Autodesk Inventor part; units mm, degrees
ref_plane "YZ Plane" through (0, 0, 0) normal (1, 0, 0) x (0, 1, 0)
ref_plane "XZ Plane" through (0, 0, 0) normal (0, 1, 0) x (-1, 0, 0)
ref_plane "XY Plane" through (0, 0, 0) normal (0, 0, 1) x (1, 0, 0)
sketch "Sketch1" plane through (0, 0, 0) normal (0, 1, 0) x (-1, 0, 0)
  line L0 (5, 7.5) -> (-5, 7.5)
  line L1 (-5, 7.5) -> (-5, -7.5)
  line L2 (-5, -7.5) -> (5, -7.5)
  line L3 (5, -7.5) -> (5, 7.5)
  point P0 (0, 0)
  dimension "d0" = 15
  dimension "d1" = 10
  dimension "d2" = 5
  dimension "d3" = 7.5
extrude "Extrusion1" add sketch "Sketch1" along normal blind 1.2
sketch "Sketch2" plane through (5, 0, 7.5) normal (1, 0, 0) x (0, 0, -1)
  line L0 (0, 0) -> (0, 1.2)
  line L1 (0, 0) -> (0, 0.8)
  line L2 (0, 0.8) -> (1.3856, 0)
  line L3 (0, 0) -> (15, 0)
  line L4 (0, 0) -> (1.3856, 0)
  line L5 (7.5, 0) -> (7.5, 5.1118)
  line L6 (15, 0) -> (15, 1.2)
  line L7 (15, 0) -> (15, 0.8)
  line L8 (15, 0.8) -> (13.6144, 0)
  line L9 (15, 0) -> (13.6144, 0)
  dimension "d6" = 0.8
  dimension "d7" = 30
extrude "Extrusion2" cut sketch "Sketch2" against normal through all
sketch "Sketch3" plane through (-5, 1.2, 7.5) normal (0, 0, 1) x (1, 0, 0)
  line L0 (0, -1.2) -> (0, -0.4)
  line L1 (0, -0.4) -> (0, -1.2)
  line L2 (0, -1.2) -> (1.3856, -1.2)
  line L3 (10, -1.2) -> (0, -1.2)
  line L4 (0, -0.4) -> (1.3856, -1.2)
  line L5 (5, -1.2) -> (5, 0.9136)
  line L6 (10, -1.2) -> (10, -0.4)
  line L7 (10, -0.4) -> (10, -1.2)
  line L8 (10, -1.2) -> (8.6144, -1.2)
  line L9 (10, -0.4) -> (8.6144, -1.2)
  dimension "d10" = 30
extrude "Extrusion3" cut sketch "Sketch3" against normal through all
properties part number "ChairTop"
The listing builds one solid part. Answer for the finished solid, in the listing's coordinates (mm). Round coordinates to 2 decimals unless told otherwise and drop trailing zeros. Write each loop counter-clockwise with the first axis right and the second up, starting at its lowest first coordinate (ties: lowest second). Pieces come first, ordered by that corner, then holes. Notation, with made-up numbers: (-15.75, -2) - (5.25, -2) arc R29 cw to (5.25, 26) - close; hole circle Ø6 at (87.5, -32). An arc over 180 degrees is marked (long way). Use a Markdown table: item, result. Add a question column.
1. Consider line 1 (X direction, y = 0.3, z = -6); line 2 (Z direction, x = 0, y = 0.4); line 3 (X direction, y = 0.5, z = -4.25). Determine where each line is inside the solid, lowest interval first.
2. The part is cut by section C-C (y = 0.3). Write down the section's boundary in (x, z).
3. The part is cut by section B-B (x = 0). Write down the section's boundary in (y, z).
4. The part is cut by section A-A (z = 5.75). Write down the section's boundary in (x, y).
Reported:
| question | item | result |
|---|---|---|
| 1 | line 1 | -4.13 to 4.13 |
| 1 | line 2 | -6.81 to 6.81 |
| 1 | line 3 | -4.48 to 4.48 |
| 2 | outline | (-4.13, -6.63) - (4.13, -6.63) - (4.13, 6.63) - (-4.13, 6.63) - close |
| 3 | outline | (0, -6.11) - (0.8, -7.5) - (1.2, -7.5) - (1.2, 7.5) - (0.8, 7.5) - (0, 6.11) - close |
| 4 | outline | (-5, 0.8) - (-3.61, 0) - (3.61, 0) - (5, 0.8) - (5, 1.2) - (-5, 1.2) - close |
